Verification items for the finished model (mm, model axes). A direction names the side the tool comes from. Give positions to 0.01 mm unless a question says otherwise; leave off trailing zeros. Write each loop counter-clockwise with the first axis right and the second up, starting at its lowest first coordinate (ties: lowest second). Pieces come first, ordered by that corner, then holes. Notation, with made-up numbers: (80, -22) -> (106, -22) arc R26 ccw to (106, -3) -> close; hole circle Ø2 at (31.25, -19.5). An arc over 180 degrees is marked (long way). Use one line per item in the form item = value. Start each with the question number.
(1) Release check for a two-part mould opening along Z. For faces 3 (the face through (5.48, -4.63, 16.16)), 4 (the face through (-17.8, 0.5, 26.6)), 5 (the face through (-3.067, -5.052, -19.59)), 6 (the face through (-5, 1, -65.848)) record: pulls with the +Z half, pulls with the -Z half, needs draft (parallel to the pull), parting line crosses it, or undercut.
(2) Set-up check for faces 1 (the face through (-2.28, -6.55, -50.29)), 2 (the face through (5.6, -34.4, 56.503)): record each of +Z, -Z, +X, -X, +Y, -Y from which the full face is reachable in a straight line by a thin tool's end or side.
(3) Scan lines: L1, parallel to Z at x = -27, y = -28.5; L2, parallel to Z at x = -4, y = 29; L3, parallel to Y at x = -9, z = 22. Record each from-to range of solid material in increasing order.
(4) Section check B-B, the plane z = 41. Record the cut outline in (x, y).
(5) Section check A-A, the plane z = -3.5. Record the cut outline in (x, y).
(6) Depth check by flat-ended pin: pin 1 Ø1 at (y, z) = (14, 22.5) entering from +X; pin 2 Ø5 at (y, z) = (1.5, -19) entering from -X; pin 3 Ø10 at (y, z) = (-6.5, -44) entering from +X. Enter the tip coordinate at first touch or a pass-through.
(7) Section check C-C, the plane z = 14. Record the cut outline in (x, y), plus the area to 3 significant figures.
from build123d import *

# Parameters (mm, degrees)
F2_R = 5.08
F3_R = 5.08


with BuildPart() as f1:
    # F0 (on Front) → F1 (revolve)
    with BuildSketch(Plane.XZ):
        Polygon((45.1151281595, 56.5034113824), (27.5946892798, 56.5034113824), (-5.6941420771, 9.4902375713), (-5.6941420771, -65.8476427197), (34.8948761821, -65.8476427197), (0, -49.4952350855), (0, 9.4902375713), align=None)
    revolve(axis=Axis((-5.6941420771, 0, -28.1787025742), (0, 0, 1)))

    # F2
    f2_edges = [f1.edges().sort_by_distance(p)[0] for p in [
        (-56.503412, 0, 56.503411),
    ]]
    fillet(f2_edges, radius=F2_R)

    # F3
    f3_edges = [f1.edges().sort_by_distance(p)[0] for p in [
        (-38.982973, 0, 56.503411),
    ]]
    fillet(f3_edges, radius=F3_R)


solid = f1.part
Completed:
q1.face_3 = undercut
q1.face_4 = pulls with the +Z half
q1.face_5 = undercut
q1.face_6 = pulls with the -Z half
q2.face_1 = none
q2.face_2 = +Z, +X, -X, +Y, -Y
q3.L1 = -65.85 to -63.5, 40.64 to 56.49
q3.L2 = -65.85 to -60.44, 33.83 to 50.52
q3.L3 = -17.39 to -8.22, 8.22 to 17.39
q4.outline = circle Ø71.86 at (-5.69, 0); hole circle Ø44.62 at (-5.69, 0)
q5.outline = circle Ø11.39 at (-5.69, 0)
q6.pin_1 = 6.83
q6.pin_2 = -11.39
q6.pin_3 = -0.2
q7.outline = circle Ø20.04 at (-5.69, 0); hole circle Ø6.39 at (-5.69, 0)
q7.area = 283 mm²
